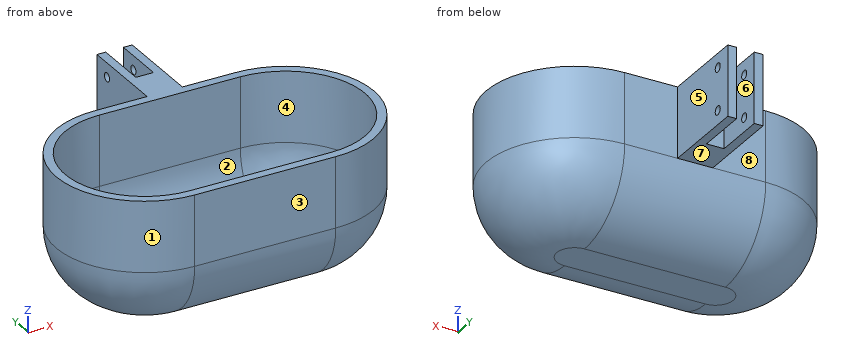
```python
from build123d import *

# Parameters (mm, degrees)
BOSS_EXTRUDE1_DEPTH          = 80
FILLET1_R                    = 40
SHELL1_T                     = -5
SKETCH3_W                    = 20
SKETCH3_H                    = 40
BOSS_EXTRUDE2_DEPTH          = 50
CUT_EXTRUDE_THIN1_DEPTH      = 215.00934559
CUT_EXTRUDE_THIN1_DEPTH_BACK = 30
SKETCH4_W                    = 10
SKETCH4_H                    = 40
SKETCH5_R                    = 2.5
CUT_EXTRUDE1_DEPTH           = 92


with BuildPart() as part:
    # Sketch2 → Boss-Extrude1 (new body)
    with BuildSketch(Plane.XY):
        with BuildLine():
            Line((0, -50), (-80, -50))
            ThreePointArc((-80, -50), (-130, 0), (-80, 50))
            Line((-80, 50), (0, 50))
            ThreePointArc((0, 50), (50, 0), (0, -50))
        make_face()
    extrude(amount=BOSS_EXTRUDE1_DEPTH)

    # Fillet1
    fillet1_edges = [part.edges().sort_by_distance(p)[0] for p in [
        (-40, -50, 0),
        (-130, 0, 0),
        (-40, 50, 0),
        (50, 0, 0),
    ]]
    fillet(fillet1_edges, radius=FILLET1_R)

    # Shell1
    shell1_openings = [part.faces().sort_by_distance(p)[0] for p in [
        (-40, 0, 80),
    ]]
    offset(amount=SHELL1_T, openings=shell1_openings, kind=Kind.INTERSECTION)

    # Sketch3 → Boss-Extrude2 (add)
    with BuildSketch(Plane(origin=(0, 50, 0), x_dir=(1, 0, 0), z_dir=(0, 1, 0))):
        with Locations((-40, -60)):
            Rectangle(SKETCH3_W, SKETCH3_H)
    extrude(amount=BOSS_EXTRUDE2_DEPTH)

    # Sketch4 → Cut-Extrude-Thin1 (cut, two sides: drawn at the far end of the back side and taken through both)
    with BuildSketch(Plane(origin=(0, 100, 0), x_dir=(1, 0, 0), z_dir=(0, 1, 0)).offset(-CUT_EXTRUDE_THIN1_DEPTH_BACK)):
        with Locations((-40, -60)):
            Rectangle(SKETCH4_W, SKETCH4_H)
    extrude(amount=CUT_EXTRUDE_THIN1_DEPTH + CUT_EXTRUDE_THIN1_DEPTH_BACK, mode=Mode.SUBTRACT)

    # Sketch5 → Cut-Extrude1 (cut)
    with BuildSketch(Plane(origin=(-30, 0, 0), x_dir=(0, 0, -1), z_dir=(1, 0, 0))):
        with Locations((-72, 90)):
            Circle(SKETCH5_R)
        with Locations((-48, 90)):
            Circle(SKETCH5_R)
    extrude(amount=-CUT_EXTRUDE1_DEPTH, mode=Mode.SUBTRACT)


solid = part.part
```
Could you check a few things on this model? Use its own coordinates, in mm. Face numbers are marked on the shaded views. A direction names the side the tool comes from. Round coordinates to 2 decimals unless told otherwise and drop trailing zeros. Loops run counter-clockwise (first coordinate to the right, second up) from the corner with the lowest first, then second, coordinate; pieces in that order, holes last. Notation, with made-up numbers: M -12,-26 L 47,-26 A30 ccw 47,0 Z; hole C 42,9 d3. An arc over 180 degrees is marked long. Answer as CSV lines item,"result".
1) If I drill on probe 1 along Y at (x, z) = (-31, 72); probe 2 along Y at (x, z) = (-74, 74.5); probe 3 along X at (y, z) = (63, 77), over which ranges is the centre line in solid material (lowest first)?
From the geometry:
probe 1,"-50 to -45, 45 to 87.5, 92.5 to 100"
probe 2,"-50 to -45, 45 to 50"
probe 3,"-50 to -30"
2) For pin 1 Ø10 at (x, y) = (-54.5, 7.5) entering from +Z; pin 2 Ø2 at (x, y) = (-49, -30.5) entering from +Z; pin 3 Ø24 at (x, z) = (-66, 54) entering from +Y, each with a flat end and sliding along its axis, tell me the tip position at first contact or that it passes through.
From the geometry:
pin 1,"z = 5.09"
pin 2,"z = 12.38"
pin 3,"y = 50"
3) Imagine slicing it at C-C on z = 59. List the corners of the cut face in (x, y) for me.
From the geometry:
outline,"M -80,-50 L 0,-50 A50 ccw 0,50 L -30,50 L -30,100 L -35,100 L -35,70 L -45,70 L -45,100 L -50,100 L -50,50 L -80,50 A50 ccw Z; hole M -80,-45 L 0,-45 A45 ccw 0,45 L -80,45 A45 ccw Z"
4) We'd pull the mould along X, two halves only. Please class the marked faces 1, 2 and 3: released by +X, released by -X, zero draft, split by the parting line, or undercut.
From the geometry:
face 1,"released by -X"
face 2,"undercut"
face 3,"zero draft"
5) Which directions (+Z, -Z, +X, -X, +Y, -Y) give clear straight access to the entire face, cutting with the end or side of a thin tool? Please do the marked faces 4, 5, 6, 7 and 8.
From the geometry:
face 4,"+Z"
face 5,"+Z, -Z, +X, +Y"
face 6,"+Z, -Z, +Y"
face 7,"-Z, +X, -X, +Y"
face 8,"+Z, -Z, -X, +Y"
6) Imagine slicing it at A-A on y = 90. List the corners of the cut face in (x, z) for me.
From the geometry:
outline,"M -50,40 L -45,40 L -45,45.5 L -50,45.5 Z; M -50,50.5 L -45,50.5 L -45,69.5 L -50,69.5 Z; M -50,74.5 L -45,74.5 L -45,80 L -50,80 Z; M -35,40 L -30,40 L -30,45.5 L -35,45.5 Z; M -35,50.5 L -30,50.5 L -30,69.5 L -35,69.5 Z; M -35,74.5 L -30,74.5 L -30,80 L -35,80 Z"
7) Imagine slicing it at B-B on z = 48. List the corners of the cut face in (x, y) for me.
From the geometry:
outline,"M -80,-50 L 0,-50 A50 ccw 0,50 L -30,50 L -30,87.5 L -35,87.5 L -35,70 L -45,70 L -45,87.5 L -50,87.5 L -50,50 L -80,50 A50 ccw Z; M -50,92.5 L -45,92.5 L -45,100 L -50,100 Z; M -35,92.5 L -30,92.5 L -30,100 L -35,100 Z; hole M -80,-45 L 0,-45 A45 ccw 0,45 L -80,45 A45 ccw Z"
